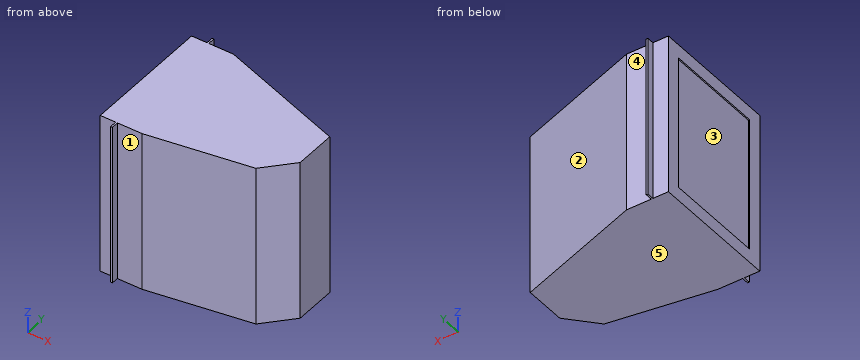
from build123d import *

# Parameters (mm, degrees)
PAD_DEPTH    = 385
SKETCH001_W  = 241
SKETCH001_H  = 320
POCKET_DEPTH = 3


with BuildPart() as part:
    # Sketch → Pad (new body)
    with BuildSketch(Plane.XY):
        Polygon((0, 0), (0, 309), (37, 309), (37, 326), (41, 326), (41, 309), (100, 309), (405, 203), (405, 103), (345, 38), (100, 0), (41, 0), (41, -17), (37, -17), (37, 0), align=None)
    extrude(amount=PAD_DEPTH)

    # Sketch001 (on Face1 of Pad) → Pocket (cut)
    with BuildSketch(Plane(origin=(0, 0, 0), x_dir=(0, -1, 0), z_dir=(-1, 0, 0))):
        with Locations((-154.5, 192.5)):
            Rectangle(SKETCH001_W, SKETCH001_H)
    extrude(amount=-POCKET_DEPTH, mode=Mode.SUBTRACT)


solid = part.part
CAD build for the part. Positions are in the model's coordinates, mm. Face numbers are marked on the shaded views. A direction names the side the tool comes from. Coordinates: 2 decimals unless noted, no trailing zeros. Loops run counter-clockwise (first coordinate to the right, second up) from the corner with the lowest first, then second, coordinate; pieces in that order, holes last. Notation, with made-up numbers: (-20, 41) - (38, 41) arc R27 ccw to (38, 71) - close; hole circle Ø4 at (-28.75, -30). An arc over 180 degrees is marked (long way). Write item = value, one per line. Start each with the question number.
Q1. Pull direction Z, two halves, no side cores. Call the marked faces 3, 4 and 5: pulls with the +Z half, pulls with the -Z half, needs draft (parallel to the pull), parting line crosses it, or undercut.
Q2. Drill centre lines: L1, parallel to Y at x = 96, z = 308.5; L2, parallel to X at y = 132, z = 311.5; L3, parallel to X at y = 82, z = 18. Where is each one in solid material? Low to high.
Q3. Which spindle directions (+Z, -Z, +X, -X, +Y, -Y) get a long thin tool onto all of the face, cutting with end or side? Do the marked faces 1 and 2. Say none if no direction does.
Q4. Cut at A-A, the plane z = 68. List the corners of the cut face in (x, y), then the cut area to 3 significant figures.
Q5. Cut at D-D, the plane x = 170. List the corners of the cut face in (y, z).
Q6. Cut at B-B, the plane x = 86. List the corners of the cut face in (y, z).
Q7. Cut at C-C, the plane y = 267. List the corners of the cut face in (x, z).
Q8. Flat gauge pins, fed straight in: pin 1 Ø5 at (y, z) = (-8, 286.5) entering from -X; pin 2 Ø1 at (y, z) = (51, 210.5) entering from -X; pin 3 Ø11 at (x, z) = (18, 204.5) entering from -Y. Where does each tip first touch, or does it go through?
Computed:
q1.face_3 = undercut
q1.face_4 = needs draft
q1.face_5 = pulls with the -Z half
q2.L1 = 0 to 309
q2.L2 = 3 to 405
q2.L3 = 0 to 385.62
q3.face_1 = +Z, -Z, +X, -Y
q3.face_2 = +Z, -Z, +X, +Y
q4.outline = (0, 0) - (37, 0) - (37, -17) - (41, -17) - (41, 0) - (100, 0) - (345, 38) - (405, 103) - (405, 203) - (100, 309) - (41, 309) - (41, 326) - (37, 326) - (37, 309) - (0, 309) - (0, 275) - (3, 275) - (3, 34) - (0, 34) - close
q4.area = 99,500 mm²
q5.outline = (10.86, 0) - (284.67, 0) - (284.67, 385) - (10.86, 385) - close
q6.outline = (0, 0) - (309, 0) - (309, 385) - (0, 385) - close
q7.outline = (0, 0) - (220.85, 0) - (220.85, 385) - (0, 385) - (0, 352.5) - (3, 352.5) - (3, 32.5) - (0, 32.5) - close
q8.pin_1 = 37
q8.pin_2 = 3
q8.pin_3 = 0
